from build123d import *

# Parameters (mm, degrees)
PAD_DEPTH            = 45
SKETCH001_R          = 38
POCKET_DEPTH         = 52.401
SKETCH005_R          = 1.8
POCKET001_DEPTH      = 38.2
SKETCH013_W          = 3
SKETCH013_H          = 26.2
PAD006_DEPTH         = 81
SKETCH014_W          = 3
SKETCH014_H          = 11.2
PAD007_DEPTH         = 81
SKETCH015_R          = 3.45
PAD008_DEPTH         = 45
SKETCH016_R          = 1.3
POCKET005_DEPTH      = 45
SKETCH017_W          = 18.3
SKETCH017_H          = 4.05
SKETCH061_R          = 3.8
POCKET021_DEPTH      = 2
SKETCH062_R          = 2
POCKET022_DEPTH      = 84.001
SKETCH064_W          = 4
SKETCH064_H          = 2
POCKET023_DEPTH      = 3
POCKET024_DEPTH      = 45.001
POCKET024_DEPTH_BACK = 45.001
POCKET029_DEPTH      = 2.9


with BuildPart() as part:
    # Sketch → Pad (new body, symmetric)
    with BuildSketch(Plane.YZ):
        Polygon((0, 84), (3, 84), (3, 3), (29.2, 3), (29.2, 84), (38.2, 84), (38.2, 3), (49.4, 3), (49.4, 84), (52.4, 84), (52.4, 0), (0, 0), align=None)
    extrude(amount=PAD_DEPTH, both=True)

    # Sketch001 → Pocket (cut, through all)
    with BuildSketch(Plane.XZ):
        with Locations((0, 43)):
            Circle(SKETCH001_R)
    extrude(amount=-POCKET_DEPTH, mode=Mode.SUBTRACT)

    # Sketch005 → Pocket001 (cut)
    with BuildSketch(Plane.XZ):
        with Locations((-35.75, 78.75)):
            Circle(SKETCH005_R)
        with Locations((35.75, 78.75)):
            Circle(SKETCH005_R)
    extrude(amount=-POCKET001_DEPTH, mode=Mode.SUBTRACT)

    # Sketch013 (on DatumPlane) → Pad006 (join)
    with BuildSketch(Plane.XY.offset(3)):
        with Locations((-43.5, 16.1)):
            Rectangle(SKETCH013_W, SKETCH013_H)
        with Locations((43.5, 16.1)):
            Rectangle(SKETCH013_W, SKETCH013_H)
    extrude(amount=PAD006_DEPTH)

    # Sketch014 (on DatumPlane) → Pad007 (join)
    with BuildSketch(Plane.XY.offset(3)):
        with Locations((-43.5, 43.8)):
            Rectangle(SKETCH014_W, SKETCH014_H)
        with Locations((43.5, 43.8)):
            Rectangle(SKETCH014_W, SKETCH014_H)
    extrude(amount=PAD007_DEPTH)

    # Sketch015 → Pad008 (join, symmetric)
    with BuildSketch(Plane.YZ):
        Circle(SKETCH015_R)
    extrude(amount=PAD008_DEPTH, both=True)

    # Sketch016 → Pocket005 (cut, symmetric)
    with BuildSketch(Plane.YZ):
        Circle(SKETCH016_R)
    extrude(amount=POCKET005_DEPTH, both=True, mode=Mode.SUBTRACT)

    # Sketch017 → Groove001 (revolve, cut)
    with BuildSketch(Plane.XZ):
        with Locations((-17.85, 2.025)):
            Rectangle(SKETCH017_W, SKETCH017_H)
        with Locations((17.85, 2.025)):
            Rectangle(SKETCH017_W, SKETCH017_H)
    revolve(axis=Axis((0, 0, 0), (1, 0, 0)), mode=Mode.SUBTRACT)

    # Sketch061 → Pocket021 (cut)
    with BuildSketch(Plane.YZ.offset(45)):
        with Locations((22.9809703886, 22.9809703886)):
            Circle(SKETCH061_R)
        with Locations((28.145825623, 16.25)):
            Circle(SKETCH061_R)
        with Locations((31.3925893544, 8.4116189658)):
            Circle(SKETCH061_R)
    extrude(amount=-POCKET021_DEPTH, mode=Mode.SUBTRACT)

    # Sketch062 → Pocket022 (cut, through all)
    with BuildSketch(Plane.XY):
        with Locations((33, 15)):
            Circle(SKETCH062_R)
    extrude(amount=POCKET022_DEPTH, mode=Mode.SUBTRACT)

    # Sketch064 → Pocket023 (cut)
    with BuildSketch(Plane.XZ):
        with Locations((40, 83)):
            Rectangle(SKETCH064_W, SKETCH064_H)
    extrude(amount=-POCKET023_DEPTH, mode=Mode.SUBTRACT)

    # Sketch065 → Pocket024 (cut, two sides)
    with BuildSketch(Plane.YZ) as pocket024_sk:
        with BuildLine():
            Line((3.45, 0), (52.4, 0))
            Line((52.4, 0), (52.4, 1))
            Line((52.4, 1), (3.3018933962, 1))
            ThreePointArc((3.45, 0), (3.4127724959, 0.5054541438), (3.3018933962, 1))
        make_face()
    extrude(amount=-POCKET024_DEPTH, mode=Mode.SUBTRACT)
    extrude(pocket024_sk.sketch, amount=POCKET024_DEPTH_BACK, mode=Mode.SUBTRACT)

    # Sketch070 (on DatumPlane) → Pocket029 (cut)
    with BuildSketch(Plane.XZ.offset(-32.2)):
        Polygon((-32.7, 76.989081679), (-32.7, 80.510918321), (-32.7, 84), (-38.8, 84), (-38.8, 80.510918321), (-38.8, 76.989081679), (-35.75, 75.2281633579), align=None)
        Polygon((38.8, 76.989081679), (38.8, 80.510918321), (38.8, 84), (32.7, 84), (32.7, 80.510918321), (32.7, 76.989081679), (35.75, 75.2281633579), align=None)
    extrude(amount=-POCKET029_DEPTH, mode=Mode.SUBTRACT)


solid = part.part
Geometry check sheet. Reference: the model listing, model coordinates, mm. A direction names the side the tool comes from. Coordinates: 2 decimals unless noted, no trailing zeros. Order: outer loops, then holes, each group sorted by start corner. A loop starts at its lowest first (then second) coordinate and runs counter-clockwise, first axis right, second up. Notation, with made-up numbers: M 13,87 L 51,87 A29 cw 51,126 Z; hole C -9,60.5 d11. An arc over 180 degrees is marked long. Use CSV: the item, a comma, the result in double quotes.
Item 1: Cross-section at A-A on x = 0. Record the cut outline in (y, z), then the cut area to 3 significant figures.
Returned:
outline,"M 0,3.45 A3.45 ccw long 3.3,1 L 52.4,1 L 52.4,5 L 49.4,5 L 49.4,3 L 38.2,3 L 38.2,5 L 29.2,5 L 29.2,3 L 3,3 L 3,5 L 0,5 Z; M 0,81 L 3,81 L 3,84 L 0,84 Z; M 29.2,81 L 38.2,81 L 38.2,84 L 29.2,84 Z; M 49.4,81 L 52.4,81 L 52.4,84 L 49.4,84 Z; hole C 0,0 d2.6"
area,"206 mm2"
Item 2: Cross-section at C-C on y = 15. Record the cut outline in (x, z).
Returned:
outline,"M -45,1 L 31,1 L 31,3 L -42,3 L -42,84 L -45,84 Z; M 35,1 L 45,1 L 45,84 L 42,84 L 42,3 L 35,3 Z"
Item 3: Mould release check, pull along Z, two halves, no side actions. Record for faces 1 (the cylindrical face through (20.43, 50.88, 75.04)), 2 (the cylindrical face through (-34.087, 36.628, 78.061)), 3 (the cylindrical face through (34.908, 15.601, 1.986)), 4 (the flat face through (40, 1, 82)): pulls with the +Z half, pulls with the -Z half, needs draft (parallel to the pull), parting line crosses it, or undercut.
Returned:
face 1,"undercut"
face 2,"undercut"
face 3,"needs draft"
face 4,"pulls with the +Z half"
Item 4: Tool access check on faces 5 (the flat face through (38, 3, 35)), 6 (the flat face through (8.7, 1, 1.2)), 7 (the cylindrical face through (20.43, 33.64, 75.04)). Record the directions out of +Z, -Z, +X, -X, +Y, -Y that give a thin tool (end or side, any length) a straight path to the whole face; none if there is none.
Returned:
face 5,"+Z"
face 6,"-Z, -Y"
face 7,"+Y, -Y"
Item 5: Gauge pin test, flat ends, axial feed: pin 1 Ø3 at (x, z) = (36, 78) entering from -Y; pin 2 Ø8 at (x, y) = (1.5, 25) entering from +Z; pin 3 Ø2 at (y, z) = (0, 0) entering from +X; pin 4 Ø6 at (x, y) = (-6.5, 8.5) entering from -Z. Record the tip position at first contact, or that the pin passes through.
Returned:
pin 1,"stops at y = 0"
pin 2,"stops at z = 3"
pin 3,"passes through"
pin 4,"stops at z = 1"
Item 6: Thickness scan on line 1 along Y through (x, z) = (37, 19.5); line 2 along X through (y, z) = (12, 22); line 3 along Z through (x, y) = (30, 34.5). Record the ranges inside material, lowest first.
Returned:
line 1,"y = 0 to 3, 29.2 to 38.2, 49.4 to 52.4"
line 2,"x = -45 to -42, 42 to 45"
line 3,"z = 1 to 19.68, 66.32 to 84"
Item 7: Cross-section at D-D on x = 13. Record the cut outline in (y, z), then the cut area to 3 significant figures.
Returned:
outline,"M 0,4.05 A4.05 cw 3.92,1 L 52.4,1 L 52.4,7.29 L 49.4,7.29 L 49.4,3 L 38.2,3 L 38.2,7.29 L 29.2,7.29 L 29.2,3 L 3,3 L 3,7.29 L 0,7.29 Z; M 0,78.71 L 3,78.71 L 3,84 L 0,84 Z; M 29.2,78.71 L 38.2,78.71 L 38.2,84 L 29.2,84 Z; M 49.4,78.71 L 52.4,78.71 L 52.4,84 L 49.4,84 Z"
area,"240 mm2"
Item 8: Cross-section at B-B on z = 43. Record the cut outline in (x, y).
Returned:
outline,"M -45,0 L -38,0 L -38,3 L -42,3 L -42,29.2 L -38,29.2 L -38,38.2 L -42,38.2 L -42,49.4 L -38,49.4 L -38,52.4 L -45,52.4 Z; M 38,0 L 45,0 L 45,52.4 L 38,52.4 L 38,49.4 L 42,49.4 L 42,38.2 L 38,38.2 L 38,29.2 L 42,29.2 L 42,3 L 38,3 Z"
